Autodesk Inventor part; units mm, degrees
ref_plane "YZ Plane" through (0, 0, 0) normal (1, 0, 0) x (0, 1, 0)
ref_plane "XZ Plane" through (0, 0, 0) normal (0, 1, 0) x (-1, 0, 0)
ref_plane "XY Plane" through (0, 0, 0) normal (0, 0, 1) x (1, 0, 0)
sketch "Sketch1" plane through (0, 0, 0) normal (0, 0, 1) x (1, 0, 0)
  line L0 (0, 0) -> (119.6, 0)
  line L1 (119.6, 0) -> (119.6, 150)
  line L2 (119.6, 150) -> (0, 150)
  line L3 (0, 150) -> (0, 0)
  dimension "d0" = 119.6
  dimension "d1" = 150
sketch "Sketch2" plane through (0, 0, 0) normal (1, 0, 0) x (0, 1, 0)
  circle A0 centre (0, 0) radius 12.5
  circle A1 centre (0, 0) radius 6.125
  line L0 (-12.5, 0) -> (12.5, 0)
  line L1 (12.5, 0) -> (12.5, 12.5)
  line L2 (12.5, 12.5) -> (-12.5, 12.5)
  line L3 (-12.5, 12.5) -> (-12.5, 0)
  circle A2 centre (150, 0) radius 12.5
  circle A3 centre (150, 0) radius 6.125
  line L4 (137.5, 0) -> (162.5, 0)
  line L5 (162.5, 0) -> (162.5, 12.5)
  line L6 (162.5, 12.5) -> (137.5, 12.5)
  line L7 (137.5, 12.5) -> (137.5, 0)
  line L8 (-12.5, 12.5) -> (-17.5, 12.5)
  line L9 (-17.5, 12.5) -> (-17.5, 0)
  line L10 (-17.5, 0) -> (-12.5, 0)
  line L11 (-12.5, 0) -> (-12.5, 12.5)
  line L12 (12.5, 12.5) -> (17.5, 12.5)
  line L13 (17.5, 12.5) -> (17.5, 0)
  line L14 (17.5, 0) -> (12.5, 0)
  line L15 (12.5, 0) -> (12.5, 12.5)
  point P0 (6.125, 0)
  point P1 (-6.125, 0)
  point P2 (150, 0)
  point P3 (12.5, 0)
  dimension "d2" = 25
  dimension "d3" = 12.25
  dimension "d6" = 5
  dimension "d7" = 5
  dimension "d8" = 35
extrude "Extrusion1" add sketch "Sketch2" along normal up to surface (119.6 mm away) contours L3 L2 A0 | A0 L0 A1 | L10 L9 L8 L3 | A0 L2 L1 | L1 L12 L13 L14 | A1 L0 picked at (10.2705, 0.9272) picked at (1.5282, 2.3311)
ref_plane "Work Plane1" through (59.8, 0, 0) normal (-1, 0, 0) x (0, 0, 1)
sketch "Sketch3" plane through (0, -17.5, 0) normal (0, -1, 0) x (1, 0, 0)
  line L0 (0, 12.5) -> (119.6, 12.5)
  line L1 (102.1, 12.5) -> (137.1, 12.5)
  line L2 (137.1, 12.5) -> (137.1, 0)
  line L3 (137.1, 0) -> (102.1, 0)
  line L4 (102.1, 0) -> (102.1, 12.5)
  line L5 (119.6, 12.5) -> (119.6, 0)
  circle A0 centre (119.6, 0) radius 8.925
  point P0 (0, 0)
  point P1 (119.6, 12.5)
  point P2 (128.525, 0)
  point P3 (110.675, 0)
  dimension "d9" = 35
  dimension "d33" = 17.85
extrude "Extrusion2" add sketch "Sketch3" against normal blind 55 contours L0 L5 A0 L3 L4 | L1 L2 L3 A0 L5 | A0 L3 L5 | L5 L3 A0
extrude "Extrusion4" cut sketch "Sketch3" along normal through all both and the other way through all contours A0 L3 L5 | L5 L3 A0
extrude "Extrusion3" cut sketch "Sketch2" along normal up to surface (119.6 mm away) contours A1 L0 picked at (1.5282, 2.3311)
mirror "Mirror1" about plane through (59.8, 0, 0) normal (-1, 0, 0) of "Extrusion2", "Extrusion4", "Extrusion3"
sketch "Sketch4" plane through (102.1, 17.5, 12.5) normal (0, 0, 1) x (1, 0, 0)
  line L0 (-119.6, -35) -> (35, -35)
  line L1 (0, 20) -> (35, 20)
  line L2 (0, 0) -> (0, 20)
  line L3 (-84.6, 0) -> (0, 0)
  line L4 (-84.6, 0) -> (-84.6, 20)
  line L5 (-84.6, 20) -> (-119.6, 20)
  line L6 (35, -35) -> (35, 20)
  line L7 (-119.6, -35) -> (-119.6, 20)
  point P0 (-102.1, -17.5)
extrude "Extrusion5" add sketch "Sketch4" along normal blind 5
sketch "Sketch5" plane through (102.1, 17.5, 0) normal (0, 0, -1) x (-1, 0, 0)
  circle A0 centre (16.425, -6.375) radius 2
  line L0 (-8.575, -11.375) -> (93.175, -11.375)
  line L1 (-8.575, 20) -> (-8.575, -11.375)
  circle A1 centre (65.675, -6.375) radius 2
  circle A2 centre (16.425, -28.625) radius 2
  circle A3 centre (65.675, -28.625) radius 2
  line L2 (93.175, -35) -> (93.175, -23.625)
  line L3 (93.175, -23.625) -> (-8.575, -23.625)
  circle A4 centre (-30, -17.5) radius 2
  circle A5 centre (117.6, -17.5) radius 2
  line L4 (-35, -35) -> (-35, 20)
  line L5 (119.6, -35) -> (119.6, 20)
  line L6 (16.425, -6.375) -> (16.425, -28.625) construction
  point P0 (102.1, -17.5)
  point P1 (16.425, -17.5)
  dimension "d18" = 4
  dimension "d19" = 5
  dimension "d20" = 25
  dimension "d23" = 49.25
  dimension "d26" = 22.25
  dimension "d29" = 27.5
  dimension "d30" = 5
  dimension "d38" = 5
  dimension "d39" = 2
extrude "Extrusion6" cut sketch "Sketch5" against normal blind 10
sketch "Sketch6" plane through (0, 37.5, 0) normal (0, 1, 0) x (1, 0, 0)
  circle A0 centre (0, 0) radius 12.325
  line L0 (-17.5, 0) -> (-17.5, -17.5)
  line L1 (-17.5, -17.5) -> (-21, -17.5)
  line L2 (-21, -17.5) -> (-21, 0)
  line L3 (-21, 0) -> (-17.5, 0)
  line L4 (-17.5, 0) -> (-17.5, -17.5)
  line L5 (-17.5, 0) -> (-8.925, 0)
  dimension "d34" = 24.65
  dimension "d40" = 3.5
extrude "Extrusion7" cut sketch "Sketch6" against normal through all contours A0
extrude "Extrusion8" add sketch "Sketch6" against normal up to surface (55 mm away) contours L0 L1 L2 L3
fillet "Fillet1" radius 2 8 edges at (102.1, 17.5, 8.75) (17.5, 17.5, 8.75) (17.5, 37.5, 8.75) (102.1, 37.5, 8.75) (137.1, 37.5, 8.75) (137.1, -17.5, 8.75) (-21, 37.5, 8.75) (-21, -17.5, 8.75)
sketch "Sketch7" plane through (-21, -15.5, 17.5) normal (-1, 0, 0) x (0, 0, 1)
  circle A0 centre (-3.7125, 10) radius 2
  line L0 (0, 51) -> (0, 0)
  line L1 (-17.5, -2) -> (0, -2)
  circle A1 centre (-3.7125, 47.75) radius 2
  point P0 (-17.5, 15.5)
  dimension "d43" = 4
  dimension "d44" = 3.7125
  dimension "d45" = 12
  dimension "d49" = 37.75
extrude "Extrusion9" cut sketch "Sketch7" against normal blind 5
extrude "Extrusion10" cut sketch "Sketch7" along normal blind 5 from surface at -158.1
equation "\"d7\" = d6"
equation "\"d9\" = d8"
properties part number "BottomBase"
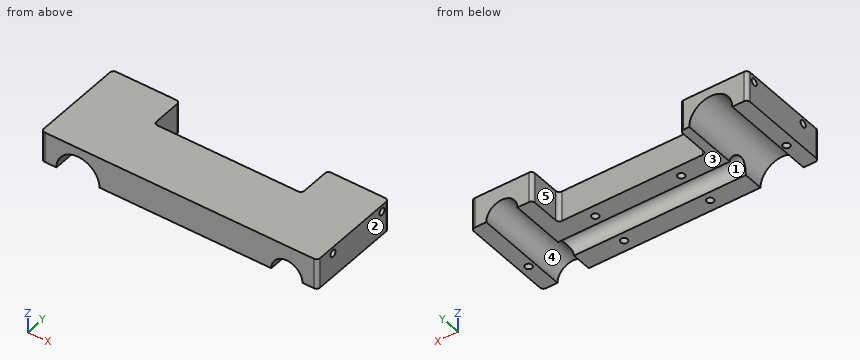
Verification items for the finished model (mm, model axes). Face numbers are marked on the shaded views. A direction names the side the tool comes from. Give positions to 0.01 mm unless a question says otherwise; leave off trailing zeros. Write each loop counter-clockwise with the first axis right and the second up, starting at its lowest first coordinate (ties: lowest second). Pieces come first, ordered by that corner, then holes. Notation, with made-up numbers: M 17.25,-16.75 L 35.25,-16.75 A26 ccw 35.25,22.25 Z; hole C 9,16.25 d3. An arc over 180 degrees is marked long. Write item = value, one per line.
(1) Access from +Z, -Z, +X, -X, +Y, -Y to the whole of each face (thin tool, end or side, straight path). Record for the marked faces 4 and 5.
Found:
face_4 = -Z, +Y, -Y
face_5 = +Z, -Z, +Y
(2) Go/stop test with flat-tipped pins: pin 1 Ø3 at (y, z) = (32.25, 13.79) entering from +X; pin 2 Ø1.2 at (x, y) = (35.5, 12) entering from -Z; pin 3 Ø9 at (x, z) = (75.5, 4.5) entering from +Y. Record where each tip stops, or that it passes through.
Found:
pin_1 = 132.1
pin_2 = 10
pin_3 = 17.5
(3) Sectioned sample at D-D (x = 0). Record the cut outline in (y, z) (3 decimals), then the cut area to 3 significant figures.
Found:
outline = M -17.5,12.325 L 37.5,12.325 L 37.5,17.5 L -17.5,17.5 Z
area = 285 mm2
(4) Draft check along X on the marked faces 1, 2 and 3. Enter one of: released by +X, released by -X, zero draft, split by the parting line, or undercut.
Found:
face_1 = undercut
face_2 = released by +X
face_3 = zero draft
(5) Sectioned sample at C-C (x = 79). Record the cut outline in (y, z) (3 decimals).
Found:
outline = M -17.5,0 L -6.125,0 A6.125 cw 6.125,0 L 17.5,0 L 17.5,17.5 L -17.5,17.5 Z
(6) Sectioned sample at B-B (z = 3.5). Give the number of separate pieces and of enclosed holes in the cut face, then the cut area to 3 significant figures.
Found:
separate_pieces = 4
enclosed_holes = 6
area = 3,720 mm2
(7) Material ranges on line 1 (X direction, y = 27, z = 9.75); line 2 (X direction, y = 27, z = 7.75); line 3 (Z direction, x = 134, y = 32), recorded low to high.
Found:
line_1 = -21 to -7.54, 7.54 to 17.5, 102.1 to 137.1
line_2 = -21 to -9.58, 9.58 to 17.5, 102.1 to 115.17, 124.03 to 137.1
line_3 = 0 to 11.8, 15.77 to 17.5
